Here's the drawing with two shaded views (mm, measured from the low corner). I have some questions. A direction names the side the tool comes from. Coordinates: 2 decimals unless noted, no trailing zeros. Write each loop counter-clockwise with the first axis right and the second up, starting at its lowest first coordinate (ties: lowest second). Pieces come first, ordered by that corner, then holes. Notation, with made-up numbers: M -29.75,-33 L -3.75,-33 A27 cw -3.75,-1 Z; hole C -30.5,33 d6. An arc over 180 degrees is marked long. Use one line per item in the form item = value. Start each with the question number.
1. I want a section at D-D, the plane y = 35.5. List the corners of the cut face in (x, z) for me, plus the area to 3 significant figures.
2. I want a section at C-C, the plane z = 77. List the corners of the cut face in (x, y) for me.
3. On a 3-axis mill with a long thin cutter (end or side, diameter ignored), from which of +Z, -Z, +X, -X, +Y, -Y can I reach the whole of each face in a straight line? I mean the marked faces 4, 5 and 6. Say none if no direction works.
4. I want a section at B-B, the plane y = 54.5. List the corners of the cut face in (x, z) for me.
5. I want a section at A-A, the plane x = 118. List the corners of the cut face in (y, z) for me.
6. Please list where these lines run through material, in increasing order: line 1 along X through (y, z) = (98, 1); line 2 along X through (y, z) = (98, 83.35); line 3 along Z through (x, y) = (26, 96). Write a range as [from, to].
7. Thinking about a two-plate mould opening in Z: for the marked faces 1, 2 and 3, which applies, released by +Z, released by -Z, zero draft, split by the parting line, or undercut?
8. I'm going to push flat-ended pins straight in: pin 1 Ø1.9 at (x, y) = (65, 98) entering from +Z; pin 2 Ø4 at (x, z) = (39.5, 72) entering from +Y; pin 3 Ø12 at (x, y) = (41, 68.5) entering from +Z. Where does each tip first touch, or does it pass through?
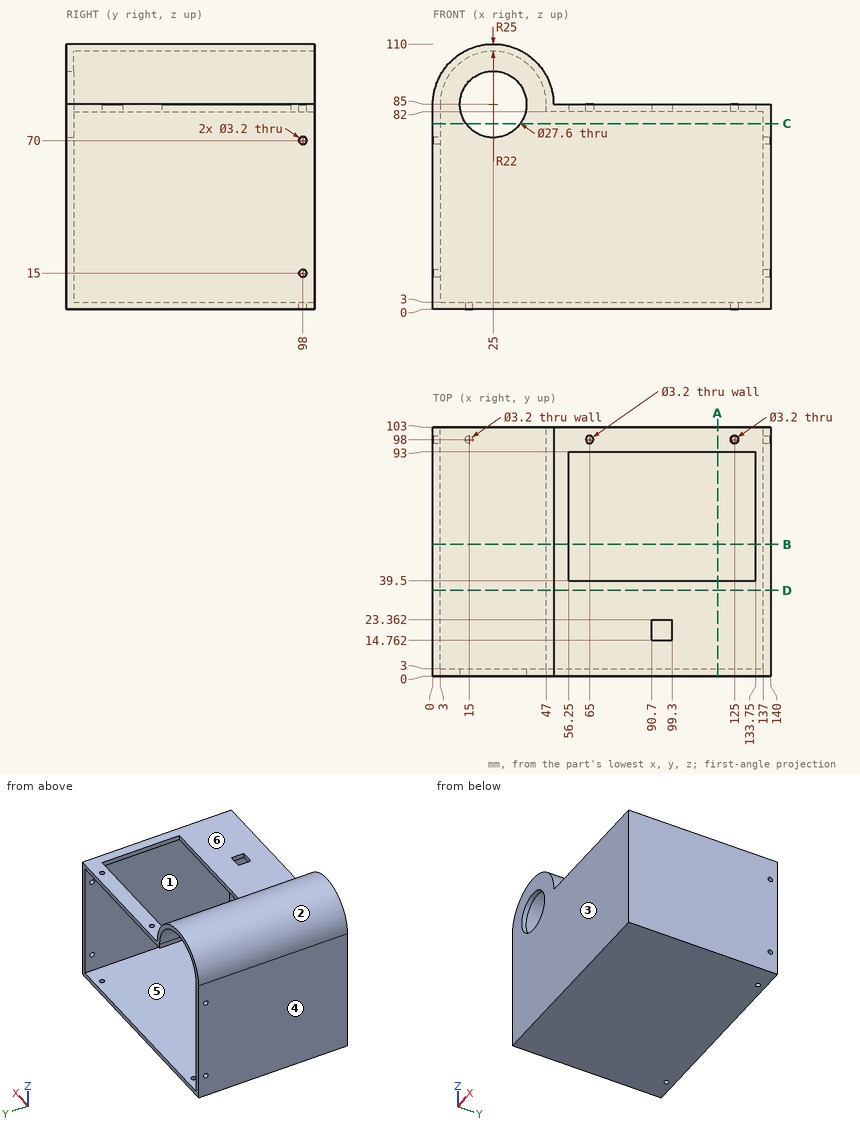
Answer list:
q1.outline = M 0,0 L 140,0 L 140,85 L 50,85 A25 ccw 0,85 Z; hole M 3,3 L 137,3 L 137,82 L 47,82 L 47,85 A22 ccw 3,85 Z
q1.area = 1,400 mm²
q2.outline = M 0,0 L 13.76,0 L 13.76,3 L 3,3 L 3,103 L 0,103 Z; M 36.24,0 L 140,0 L 140,103 L 137,103 L 137,3 L 36.24,3 Z
q3.face_4 = +Z, -Z, -X, +Y, -Y
q3.face_5 = +Y
q3.face_6 = +Z, +X, +Y, -Y
q4.outline = M 0,0 L 140,0 L 140,85 L 133.75,85 L 133.75,82 L 137,82 L 137,3 L 3,3 L 3,85 A22 cw 47,85 L 47,82 L 56.25,82 L 56.25,85 L 50,85 A25 ccw 0,85 Z
q5.outline = M 0,0 L 103,0 L 103,3 L 3,3 L 3,82 L 39.5,82 L 39.5,85 L 0,85 Z; M 93,82 L 103,82 L 103,85 L 93,85 Z
q6.line_1 = [0, 13.4], [16.6, 123.4], [126.6, 140]
q6.line_2 = [0, 3], [47, 63.4], [66.6, 123.4], [126.6, 140]
q6.line_3 = [0, 3], [106.98, 109.98]
q7.face_1 = undercut
q7.face_2 = released by +Z
q7.face_3 = zero draft
q8.pin_1 = 3
q8.pin_2 = 3
q8.pin_3 = 107.91
